Could you check a few things on this drawing? It's one solid part, dimensions in mm from its lowest x, y, z. A direction names the side the tool comes from. Give positions to 0.01 mm unless a question says otherwise; leave off trailing zeros. Loops run counter-clockwise (first coordinate to the right, second up) from the corner with the lowest first, then second, coordinate; pieces in that order, holes last.
Q1. I need wall thicknesses on probe 1 along Z at (x, y) = (49.5, 19); probe 2 along Y at (x, z) = (55, 22); probe 3 along X at (y, z) = (24, 32). Which ranges of each line are inside material? Lowest first, please.
Q2. For the marked faces 1, 2, 3 and 4, which set-ups out of +Z, -Z, +X, -X, +Y, -Y let a thin tool reach every point of the face, with its end or its side?
Q3. I'm going to push flat-ended pins straight in: P1, Ø22, axis at x = 11, y = 5.5, coming from the +Z side; P2, Ø3, axis at x = 80.5, y = 44.5, coming from the +Z side; P3, Ø4, axis at x = 9.5, z = 24.5, coming from the -Y side. Where does each tip first touch, or does it pass through?
Q4. Suppose I cut it at B-B (x = 18). List the corners of the cut face in (y, z) for me.
Q5. Suppose I cut it at A-A (y = 35). List the corners of the cut face in (x, z) for me, and give its area (3 significant figures).
Q6. Suppose I cut it at D-D (z = 32.5). List the corners of the cut face in (x, y) for me, and give its area (3 significant figures).
Q7. Suppose I cut it at C-C (z = 7). List the corners of the cut face in (x, y) for me, and give its area (3 significant figures).
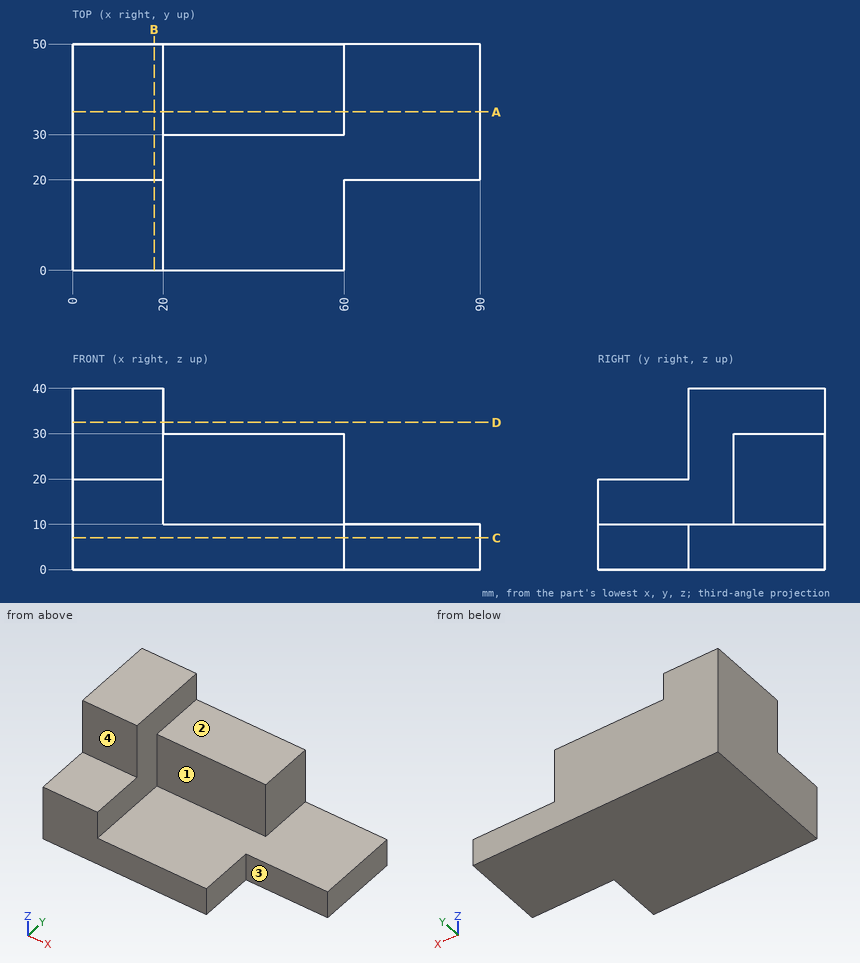
Solutions:
1. probe 1: z = 0 to 10
1. probe 2: y = 30 to 50
1. probe 3: x = 0 to 20
2. face 1: +Z, +X, -Y
2. face 2: +Z, +X, +Y, -Y
2. face 3: +Z, -Z, +X, -Y
2. face 4: +Z, +X, -X, -Y
3. P1: stops at z = 20
3. P2: stops at z = 10
3. P3: stops at y = 20
4. outline: (0, 0) - (50, 0) - (50, 40) - (20, 40) - (20, 20) - (0, 20) - close
5. outline: (0, 0) - (90, 0) - (90, 10) - (60, 10) - (60, 30) - (20, 30) - (20, 40) - (0, 40) - close
5. area: 2,300 mm2
6. outline: (0, 20) - (20, 20) - (20, 50) - (0, 50) - close
6. area: 600 mm2
7. outline: (0, 0) - (60, 0) - (60, 20) - (90, 20) - (90, 50) - (0, 50) - close
7. area: 3,900 mm2
